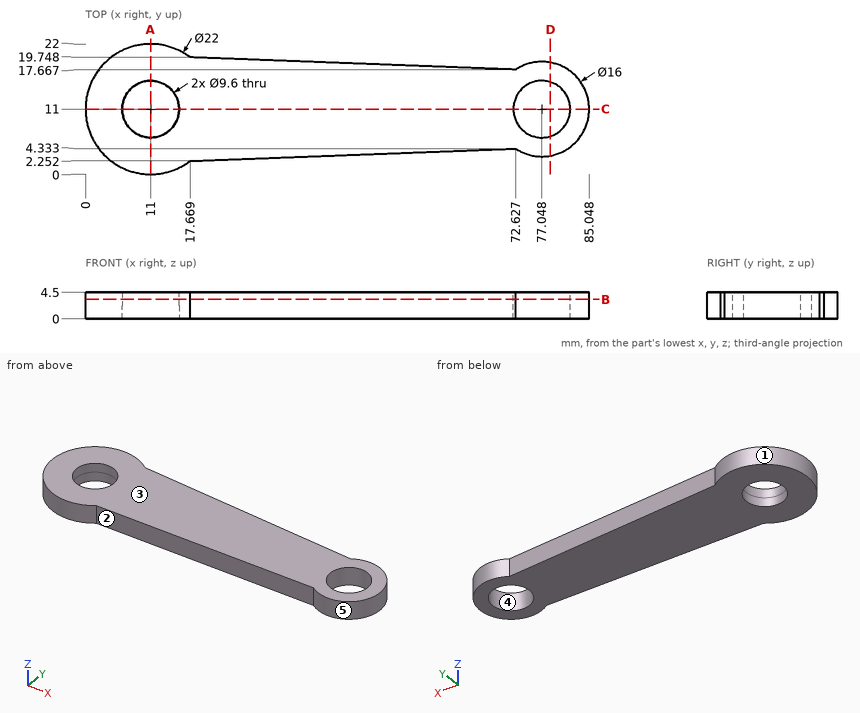
Design review of the part shown in the three views and the two pictorial views. Dimensions are in mm from the part's minimum x, y and z. A direction names the side the tool comes from. Give positions to 0.01 mm unless a question says otherwise; leave off trailing zeros. Write each loop counter-clockwise with the first axis right and the second up, starting at its lowest first coordinate (ties: lowest second). Pieces come first, ordered by that corner, then holes. Notation, with made-up numbers: M 25.25,44 L 63.25,44 A20 cw 63.25,53 Z; hole C 46.5,89.5 d5. An arc over 180 degrees is marked long. Answer as CSV lines item,"result".
1. Consider section D-D, the plane x = 78.5. Write out the cut boundary in (y, z) (1 decimal).
Findings:
outline,"M 3.1,0 L 6.4,0 L 6.4,4.5 L 3.1,4.5 Z; M 15.6,0 L 18.9,0 L 18.9,4.5 L 15.6,4.5 Z"
2. For the marked faces 1 and 2, list the 3-axis set-ups (+Z, -Z, +X, -X, +Y, -Y) from which the entire face can be reached by the end or side of a thin tool; tool diameter is ignored.
Findings:
face 1,"+Z, -Z"
face 2,"+Z, -Z, -Y"
3. Consider section B-B, the plane z = 3.3. Write out the cut boundary in (x, y), then the cut area to 3 significant figures.
Findings:
outline,"M 17.67,2.25 L 72.63,4.33 A8 ccw long 72.63,17.67 L 17.67,19.75 A11 ccw long Z; hole C 11,11 d9.6; hole C 77.05,11 d9.6"
area,"1,200 mm2"
4. Draft analysis for pull direction Y (two halves, no side actions). For the marked faces 3, 4 and 5, state which applies: +Y half, -Y half, draft (parallel to the pull), parting line (faces both ways), or undercut.
Findings:
face 3,"draft"
face 4,"undercut"
face 5,"parting line"
5. Consider section C-C, the plane y = 11. Write out the cut boundary in (x, z).
Findings:
outline,"M 0,0 L 6.2,0 L 6.2,4.5 L 0,4.5 Z; M 15.8,0 L 72.25,0 L 72.25,4.5 L 15.8,4.5 Z; M 81.85,0 L 85.05,0 L 85.05,4.5 L 81.85,4.5 Z"
6. For pin 1 (1 mm diameter, centred on x = 50.5, z = 3.5, fed in from -Y); pin 2 (1.5 mm diameter, centred on x = 47, z = 1, fed in from +Y), all flat-tipped, find the tip position at first contact; note any pin that passes through.
Findings:
pin 1,"stops at y = 3.48"
pin 2,"stops at y = 18.67"
7. Consider section A-A, the plane x = 11. Write out the cut boundary in (y, z), then the cut area to 3 significant figures.
Findings:
outline,"M 0,0 L 6.2,0 L 6.2,4.5 L 0,4.5 Z; M 15.8,0 L 22,0 L 22,4.5 L 15.8,4.5 Z"
area,"55.8 mm2"
8. Wall thickness on line 1 (X direction, y = 8, z = 1.45) (1 decimal); line 2 (Y direction, x = 11, z = 3.05); line 3 (X direction, y = 12, z = 0.45) (1 decimal): over which ranges is each line inside the solid? List them lowest first.
Findings:
line 1,"x = 0.4 to 7.3, 14.7 to 73.3, 80.8 to 84.5"
line 2,"y = 0 to 6.2, 15.8 to 22"
line 3,"x = 0 to 6.3, 15.7 to 72.4, 81.7 to 85"
